The listing builds one solid part. Answer for the finished solid, in the listing's coordinates (mm). A direction names the side the tool comes from. Give positions to 0.01 mm unless a question says otherwise; leave off trailing zeros. Write each loop counter-clockwise with the first axis right and the second up, starting at its lowest first coordinate (ties: lowest second). Pieces come first, ordered by that corner, then holes. Notation, with made-up numbers: M 35,40.5 L 74,40.5 A14 ccw 74,64.5 Z; hole C 32.25,58.5 d7. An arc over 180 degrees is marked long. Return JSON: item names as keys, results as strings.
Autodesk Inventor part; units mm, degrees
ref_plane "YZ Plane" through (0, 0, 0) normal (1, 0, 0) x (0, 1, 0)
ref_plane "XZ Plane" through (0, 0, 0) normal (0, 1, 0) x (-1, 0, 0)
ref_plane "XY Plane" through (0, 0, 0) normal (0, 0, 1) x (1, 0, 0)
sketch "Sketch1" plane through (0, 0, 0) normal (0, 0, 1) x (1, 0, 0)
  line L0 (0, 0) -> (0, 6.35)
  line L1 (0, 6.35) -> (-3.175, 6.35)
  line L2 (-3.175, 6.35) -> (-3.175, -3.175)
  line L3 (0, 0) -> (15.875, 0)
  line L4 (15.875, 0) -> (15.875, 6.35)
  line L5 (15.875, 6.35) -> (19.05, 6.35)
  line L6 (19.05, 6.35) -> (19.05, -3.175)
  line L7 (-3.175, -3.175) -> (-3.175, -19.05)
  line L8 (-3.175, -19.05) -> (19.05, -19.05)
  line L9 (19.05, -19.05) -> (19.05, -3.175)
  dimension "d0" = 6.35
  dimension "d1" = 3.175
  dimension "d2" = 9.525
  dimension "d3" = 15.875
  dimension "d4" = 3.175
  dimension "d6" = 15.875
extrude "Plate1" add sketch "Sketch1" along normal blind 3.048
sketch "Sketch2" plane through (19.05, -16.002, 0) normal (0, -1, 0) x (1, 0, 0)
  line L0 (-22.225, 0) -> (0, 0)
  line L1 (0, 0) -> (0, 25.4)
  line L2 (0, 25.4) -> (-22.225, 25.4)
  line L3 (-22.225, 25.4) -> (-22.225, 0)
edge flange "Flange1" height 25.4 angle 90 thickness 3.048 bend radius 1.27 thickness toward (0, -1, 0) relief tear relief width 3.048 relief depth 1.524 edges at (7.9375, -19.05, 3.048) wall of the first edge with corners at (-3.175, -16.002, 0) (19.05, -16.002, 0) (19.05, -16.002, 25.4) (-3.175, -16.002, 25.4)
bend "Bend1"
corner "Corner1"
sketch "Sketch3" plane through (-3.175, -16.002, 25.4) normal (0, 1, 0) x (1, 0, 0)
  line L0 (0, 0) -> (0, 21.082)
  line L1 (0, 0) -> (22.225, 0)
  line L2 (22.225, 0) -> (22.225, 21.082)
  circle A0 centre (6.35, 12.7) radius 3.3782
  circle A1 centre (15.875, 12.7) radius 3.3782
  point P0 (3.175, 25.4)
  dimension "d23" = 6.7564
  dimension "d24" = 6.7564
  dimension "d25" = 12.7
  dimension "d26" = 12.7
  dimension "d27" = 6.35
  dimension "d28" = 6.35
extrude "Cut1" cut sketch "Sketch3" against normal blind 3.048
equation "\"d29\" = Thickness"
equation "\"d13\" = BendReliefWidth"
equation "\"d14\" = BendReliefDepth"
equation "\"d15\" = MinimumRemnant"
equation "\"d16\" = BendRadius"
equation "\"d20\" = CornerReliefSize"
equation "\"d21\" = GapSize"
equation "\"d22\" = JacobiRadiusSize"
equation "\"BendRadius\" = Thickness"
equation "\"BendReliefWidth\" = Thickness"
equation "\"BendReliefDepth\" = 0.5 * Thickness"
equation "\"CornerReliefSize\" = 4 * Thickness"
equation "\"MinimumRemnant\" = 2 * Thickness"
equation "\"TransitionRadius\" = BendRadius"
equation "\"JacobiRadiusSize\" = BendRadius"
equation "\"GapSize\" = Thickness"
equation "\"d12\" = BendRadius"
properties part number "Glider"
Item 1: Find the intervals of material crossed by line 1 (X direction, y = -18.15, z = 12.7) (3 decimals); line 2 (Z direction, x = 1.5, y = -2.25); line 3 (Y direction, x = -1.75, z = 15.25), in increasing order.
Geometry results:
{"line 1": "x = -3.175 to -0.203, 6.553 to 9.322, 16.078 to 19.05", "line 2": "z = 0 to 3.05", "line 3": "y = -19.05 to -16"}
Item 2: Given pin 1 Ø9 at (x, z) = (12.7, 12.7) entering from -Y; pin 2 Ø10.5 at (x, z) = (7.5, 14.5) entering from +Y; pin 3 Ø10 at (y, z) = (-8.5, 17) entering from -X; pin 4 Ø3 at (x, y) = (13, -11) entering from +Z, each flat-ended and moving along its own axis, determine where each tip first touches the part or whether it passes through.
Geometry results:
{"pin 1": "stops at y = -19.05", "pin 2": "stops at y = -16", "pin 3": "passes through", "pin 4": "stops at z = 3.05"}
Item 3: A cutting plane is placed at B-B, the plane y = 4.5. Write down the section's boundary in (x, z) (3 decimals), plus the area to 3 significant figures.
Geometry results:
{"outline": "M -3.175,0 L 0,0 L 0,3.048 L -3.175,3.048 Z; M 15.875,0 L 19.05,0 L 19.05,3.048 L 15.875,3.048 Z", "area": "19.4 mm2"}
Item 4: Determine the mould class of faces 1 (the flat face through (-3.175, -12, 2)), 2 (the flat face through (8, -16.002, 15)), 3 (the flat face through (0, 3, 2)) for opening direction X: +X half, -X half, draft (parallel to the pull), parting line (faces both ways), or undercut.
Geometry results:
{"face 1": "-X half", "face 2": "draft", "face 3": "undercut"}
Item 5: Which of the six approach directions +Z, -Z, +X, -X, +Y, -Y give full straight-line access (tool end or side, diameter ignored) to faces 4 (the flat face through (8, -6, 3.048)), 5 (the flat face through (15.875, 3, 2)), 6 (the flat face through (-2, 6.35, 2))?
Geometry results:
{"face 4": "+Z, +X, -X, +Y", "face 5": "+Z, -Z, +Y", "face 6": "+Z, -Z, +X, -X, +Y"}
Item 6: A cutting plane is placed at C-C, the plane z = 12.7. Write down the section's boundary in (x, y) (3 decimals).
Geometry results:
{"outline": "M -3.175,-19.05 L -0.203,-19.05 L -0.203,-16.002 L -3.175,-16.002 Z; M 6.553,-19.05 L 9.322,-19.05 L 9.322,-16.002 L 6.553,-16.002 Z; M 16.078,-19.05 L 19.05,-19.05 L 19.05,-16.002 L 16.078,-16.002 Z"}
Item 7: A cutting plane is placed at A-A, the plane x = 12.7. Write down the section's boundary in (y, z).
Geometry results:
{"outline": "M -19.05,4.32 A4.32 ccw -14.73,0 L 0,0 L 0,3.05 L -14.73,3.05 A1.27 cw -16,4.32 L -16,9.32 L -19.05,9.32 Z; M -19.05,16.08 L -16,16.08 L -16,25.4 L -19.05,25.4 Z"}
Item 8: A cutting plane is placed at D-D, the plane x = 7.25. Write down the section's boundary in (y, z).
Geometry results:
{"outline": "M -19.05,4.32 A4.32 ccw -14.73,0 L 0,0 L 0,3.05 L -14.73,3.05 A1.27 cw -16,4.32 L -16,25.4 L -19.05,25.4 Z"}
